Read the model definition and answer for the solid it produces. Units are mm, in the model's axes. A direction names the side the tool comes from. Coordinates: 2 decimals unless noted, no trailing zeros. Write each loop counter-clockwise with the first axis right and the second up, starting at its lowest first coordinate (ties: lowest second). Pieces come first, ordered by that corner, then holes. Notation, with made-up numbers: (-31, -27) -> (7, -27) arc R18 cw to (7, -22) -> close; hole circle Ø8 at (33.5, 60). An arc over 180 degrees is marked (long way). One line per item, written item: value. Start each with the question number.
1. For faces 4 (the flat face through (-31.942, 0, 19)), 5 (the cylindrical face through (20.258, -15.634, 3.131)), 6 (the flat face through (-35, 0, 31.75)), 7 (the flat face through (-3, 25.4, 16)), 8 (the flat face through (3.175, 0, 28)), determine the directions among +Z, -Z, +X, -X, +Y, -Y from which every point of the face is accessible in a straight line to the end or side of a thin tool.
2. Find section A-A, the plane z = 28. Write down the section's boundary in (x, y) (3 decimals), and give its area (3 significant figures).
3. Consider line 1 along X through (y, z) = (12.5, 29) (3 decimals); line 2 along X through (y, z) = (-4, 34) (3 decimals); line 3 along Z through (x, y) = (23.5, -4.5). Determine where each line is inside the solid, lowest interval first.
4. Find section D-D, the plane z = 45. Write down the section's boundary in (x, y) (3 decimals).
5. Find section B-B, the plane y = -21. Write down the section's boundary in (x, z) (3 decimals).
6. For a pull along Y with two mould halves and no side action, classify faces 1 (the flat face through (-3, -25.4, 16)), 2 (the cylindrical face through (26.834, 13.649, 3.131)), 3 (the flat face through (20, 0, 6.35)) as pulls with the +Y half, pulls with the -Y half, needs draft (parallel to the pull), parting line crosses it, or undercut.
7. Given P1, Ø7.5, axis at y = -3, z = 25, coming from the +X side (3 decimals); P2, Ø2, axis at x = 21.5, y = 15.5, coming from the +Z side; P3, Ø6, axis at x = 0.5, y = 9, coming from the -Z side; P4, Ø7, axis at x = -34, y = -1, coming from the +Z side, each flat-ended and moving along its own axis, determine where each tip first touches the part or whether it passes through.
8. Find section C-C, the plane x = 32.5. Write down the section's boundary in (y, z), and give its area (3 significant figures).
```python
from build123d import *

# Parameters (mm, degrees)
F0_W     = 76.2
F0_H     = 50.8
F1_DEPTH = 6.35
F2_W     = 6.35
F2_H     = 50.8
F3_DEPTH = 50.8
F5_D     = 5.5
F6_W     = 6.1577814579
F6_H     = 50.8
F7_DEPTH = 25.4


with BuildPart() as f1:
    # F0 (on Top) → F1 (new body)
    with BuildSketch(Plane.XY):
        Rectangle(F0_W, F0_H)
    extrude(amount=F1_DEPTH)

    # F2 (on Top) → F3 (join)
    with BuildSketch(Plane.XY):
        Rectangle(F2_W, F2_H)
    extrude(amount=F3_DEPTH)

    # F5 (through all)
    with Locations(Plane.XY.offset(6.35)):
        with Locations((-21.0682712495, 12.8510268405), (-20.8211354911, -15.3223779052), (22.798217833, -14.5809724927), (24.6517322958, 15.3223788366)):
            Hole(F5_D / 2)

    # F6 (on face) → F7 (join)
    with BuildSketch(Plane.XY.offset(6.35)):
        with Locations((-35.021109271, 0)):
            Rectangle(F6_W, F6_H)
    extrude(amount=F7_DEPTH)


solid = f1.part
```
Answer block:
1. face 4: +Z, +Y, -Y
1. face 5: +Z, -Z
1. face 6: +Z, -X, +Y, -Y
1. face 7: +Z, -Z, +X, -X, +Y
1. face 8: +Z, +X, +Y, -Y
2. outline: (-38.1, -25.4) -> (-31.942, -25.4) -> (-31.942, 25.4) -> (-38.1, 25.4) -> close; (-3.175, -25.4) -> (3.175, -25.4) -> (3.175, 25.4) -> (-3.175, 25.4) -> close
2. area: 635 mm2
3. line 1: x = -38.1 to -31.942, -3.175 to 3.175
3. line 2: x = -3.175 to 3.175
3. line 3: z = 0 to 6.35
4. outline: (-3.175, -25.4) -> (3.175, -25.4) -> (3.175, 25.4) -> (-3.175, 25.4) -> close
5. outline: (-38.1, 0) -> (38.1, 0) -> (38.1, 6.35) -> (3.175, 6.35) -> (3.175, 50.8) -> (-3.175, 50.8) -> (-3.175, 6.35) -> (-31.942, 6.35) -> (-31.942, 31.75) -> (-38.1, 31.75) -> close
6. face 1: pulls with the -Y half
6. face 2: undercut
6. face 3: needs draft
7. P1: stops at x = 3.175
7. P2: stops at z = 6.35
7. P3: stops at z = 0
7. P4: stops at z = 31.75
8. outline: (-25.4, 0) -> (25.4, 0) -> (25.4, 6.35) -> (-25.4, 6.35) -> close
8. area: 323 mm2
